from build123d import *

# Parameters (mm, degrees)
SKETCH1_R           = 30
BOSS_EXTRUDE1_DEPTH = 10
SKETCH4_R           = 24
BOSS_EXTRUDE2_DEPTH = 6
SKETCH5_R           = 22
CUT_EXTRUDE2_DEPTH  = 11
BOSS_EXTRUDE5_DEPTH = 2
SKETCH10_R          = 30
CUT_EXTRUDE3_DEPTH  = 3


with BuildPart() as part:
    # Sketch1 → Boss-Extrude1 (new body)
    with BuildSketch(Plane(origin=(0, 0, 0), x_dir=(1, 0, 0), z_dir=(0, 1, 0))):
        with Locations(Location((0, 0, 0), (0, 0, 270))):
            Circle(SKETCH1_R)
    extrude(amount=BOSS_EXTRUDE1_DEPTH)

    # Sketch4 → Boss-Extrude2 (add)
    with BuildSketch(Plane(origin=(0, 10, 0), x_dir=(1, 0, 0), z_dir=(0, 1, 0))):
        with Locations(Location((0, 0, 0), (0, 0, 270))):
            Circle(SKETCH4_R)
    extrude(amount=BOSS_EXTRUDE2_DEPTH)

    # Sketch5 → Cut-Extrude2 (cut)
    with BuildSketch(Plane(origin=(0, 16, 0), x_dir=(1, 0, 0), z_dir=(0, 1, 0))):
        with Locations(Location((0, 0, 0), (0, 0, 270))):
            Circle(SKETCH5_R)
    extrude(amount=-CUT_EXTRUDE2_DEPTH, mode=Mode.SUBTRACT)

    # Sketch9 → Boss-Extrude5 (add)
    with BuildSketch(Plane(origin=(0, 16, 0), x_dir=(1, 0, 0), z_dir=(0, 1, 0))):
        Polygon((0.5, -23), (-2, -23), (-1.900803743, -27), (3, -27), (3, -23), align=None)
        Polygon((-3, 23), (-3, 27), (1.900803743, 27), (2, 23), (-0.5, 23), align=None)
    extrude(amount=-BOSS_EXTRUDE5_DEPTH)

    # Sketch10 → Cut-Extrude3 (cut)
    with BuildSketch(Plane.XZ):
        with Locations(Location((0, 0, 0), (0, 0, 270))):
            Circle(SKETCH10_R)
    extrude(amount=-CUT_EXTRUDE3_DEPTH, mode=Mode.SUBTRACT)


solid = part.part
Verification items for the finished model (mm, model axes). A direction names the side the tool comes from. Coordinates: 2 decimals unless noted, no trailing zeros. Loops run counter-clockwise (first coordinate to the right, second up) from the corner with the lowest first, then second, coordinate; pieces in that order, holes last. Notation, with made-up numbers: M -32,30 L 2,30 A12 cw 2,35 Z; hole C 42,68 d8. An arc over 180 degrees is marked long. One line per item, written item: value.
1. Section check C-C on y = 8.25. Record the cut outline in (x, z).
Answers follow:
outline: C 0,0 d60; hole C 0,0 d44
2. Section check D-D on z = -19. Record the cut outline in (x, y), plus the area to 3 significant figures.
Answers follow:
outline: M -23.22,3 L 23.22,3 L 23.22,10 L 14.66,10 L 14.66,16 L 11.09,16 L 11.09,5 L -11.09,5 L -11.09,16 L -14.66,16 L -14.66,10 L -23.22,10 Z
area: 257 mm^2
3. Gauge pin test, flat ends, axial feed: P1, Ø0.6, axis at x = -1, y = 15.5, coming from the -Z side; P2, Ø2, axis at x = -0.5, y = 15, coming from the +Z side; P3, Ø1.6, axis at y = 15, z = -25, coming from the -X side; P4, Ø1.5, axis at x = 23, z = 22.5, coming from the -Y side. Record the tip position at first contact, or that the pin passes through.
Answers follow:
P1: z = -27
P2: z = 27
P3: x = -3
P4: through
4. Section check B-B on z = 0. Record the cut outline in (x, y).
Answers follow:
outline: M -30,3 L 30,3 L 30,10 L 24,10 L 24,16 L 22,16 L 22,5 L -22,5 L -22,16 L -24,16 L -24,10 L -30,10 Z
5. Material ranges on line 1 along X through (y, z) = (10.25, 0); line 2 along Y through (x, z) = (-25, 12); line 3 along Z through (x, y) = (-3, 13), recorded low to high. Write a range as from..to.
Answers follow:
line 1: -24..-22, 22..24
line 2: 3..10
line 3: -23.81..-21.79, 21.79..23.81
6. Set-up check for faces 1 (the flat face through (3, 15, 25)), 2 (the cylindrical face through (-21.477, 10.577, -4.769)), 3 (the flat face through (1, 15, 27)): record each of +Z, -Z, +X, -X, +Y, -Y from which the full face is reachable in a straight line by a thin tool's end or side.
Answers follow:
face 1: +Z, +X, +Y
face 2: +Y
face 3: +Z, +X, -X, +Y
7. Section check A-A on x = 0. Record the cut outline in (y, z).
Answers follow:
outline: M 3,-30 L 10,-30 L 10,-24 L 14,-24 L 14,-27 L 16,-27 L 16,-22 L 5,-22 L 5,22 L 16,22 L 16,27 L 14,27 L 14,24 L 10,24 L 10,30 L 3,30 Z
8. Mould release check, pull along X, two halves, no side actions. Record for faces 4 (the flat face through (0, 5, 0)), 5 (the flat face through (-3, 15, -25)), 6 (the flat face through (-1, 15, -27)): pulls with the +X half, pulls with the -X half, needs draft (parallel to the pull), parting line crosses it, or undercut.
Answers follow:
face 4: undercut
face 5: pulls with the -X half
face 6: needs draft
